Geometry: see drawing. Coordinates: mm, zero at the bounding-box minimum. A direction names the side the tool comes from. Give positions to 0.01 mm unless a question says otherwise; leave off trailing zeros. Loops run counter-clockwise (first coordinate to the right, second up) from the corner with the lowest first, then second, coordinate; pieces in that order, holes last. Notation, with made-up numbers: (56.25, 46) - (86.25, 46) arc R27 cw to (86.25, 82) - close; hole circle Ø5 at (50, 34.5). An arc over 180 degrees is marked (long way). Use one line per item in the form item = value.
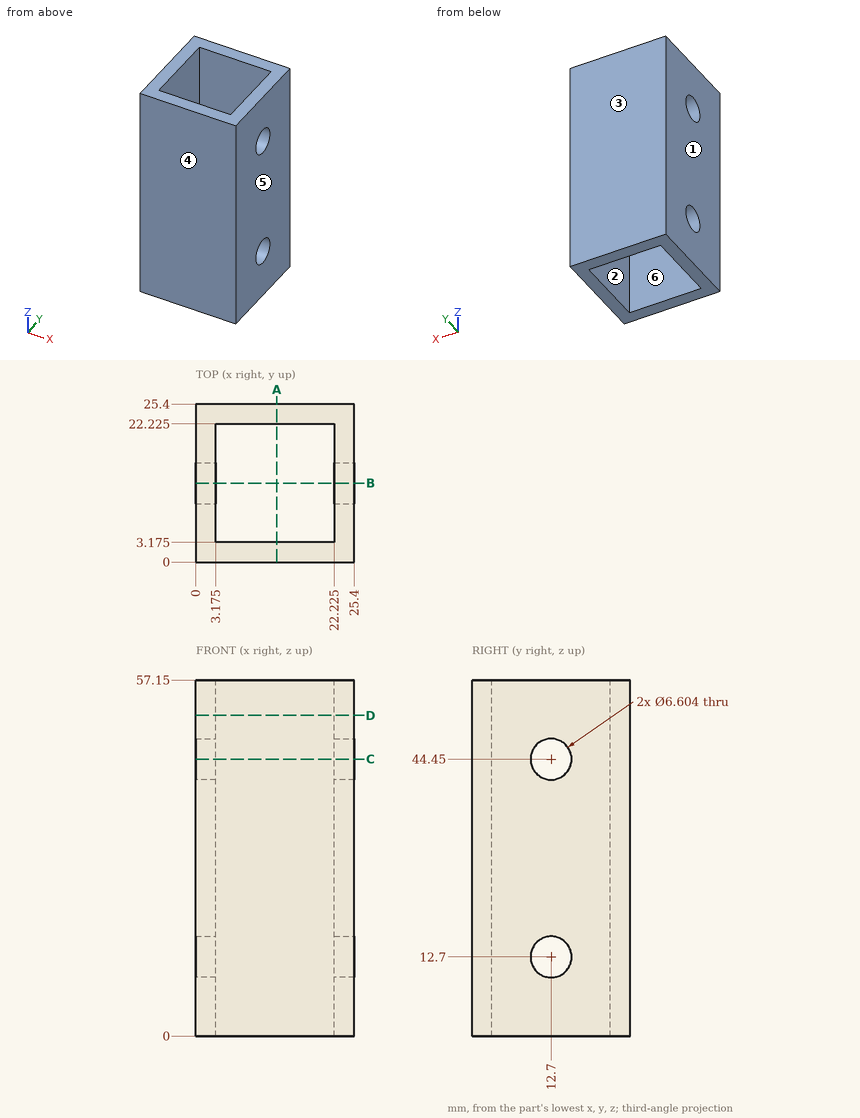
(1) Cut plane B-B (y = 12.7). Return the cut outline in (x, z) (3 decimals).
Solution:
outline = (0, 0) - (3.175, 0) - (3.175, 9.398) - (0, 9.398) - close; (0, 16.002) - (3.175, 16.002) - (3.175, 41.148) - (0, 41.148) - close; (0, 47.752) - (3.175, 47.752) - (3.175, 57.15) - (0, 57.15) - close; (22.225, 0) - (25.4, 0) - (25.4, 9.398) - (22.225, 9.398) - close; (22.225, 16.002) - (25.4, 16.002) - (25.4, 41.148) - (22.225, 41.148) - close; (22.225, 47.752) - (25.4, 47.752) - (25.4, 57.15) - (22.225, 57.15) - close
(2) Access query for the marked faces 5 and 6. Directions: +Z, -Z, +X, -X, +Y, -Y. A direction counts if a zero-diameter tool reaches every point of the face in a straight line with its end or side. Return the directions, or none.
Solution:
face_5 = +Z, -Z, +X, +Y, -Y
face_6 = +Z, -Z
(3) Cut plane A-A (x = 13). Return the cut outline in (y, z) (3 decimals), plus the area to 3 significant figures.
Solution:
outline = (0, 0) - (3.175, 0) - (3.175, 57.15) - (0, 57.15) - close; (22.225, 0) - (25.4, 0) - (25.4, 57.15) - (22.225, 57.15) - close
area = 363 mm2
(4) Material intervals for L1, parallel to Y at x = 16.5, z = 4 (3 decimals); L2, parallel to Y at x = 2.3, z = 12.7, sorted ascending. Write a range as from..to.
Solution:
L1 = 0..3.175, 22.225..25.4
L2 = 0..9.4, 16..25.4
(5) Cut plane C-C (z = 44.45). Return the cut outline in (x, y) (3 decimals).
Solution:
outline = (0, 0) - (25.4, 0) - (25.4, 9.398) - (22.225, 9.398) - (22.225, 3.175) - (3.175, 3.175) - (3.175, 9.398) - (0, 9.398) - close; (0, 16.002) - (3.175, 16.002) - (3.175, 22.225) - (22.225, 22.225) - (22.225, 16.002) - (25.4, 16.002) - (25.4, 25.4) - (0, 25.4) - close
(6) Pull-direction query (Y, two-part tool) for the marked faces 1, 2, 3 and 4; classes: released by +Y, released by -Y, zero draft, split by the parting line, or undercut.
Solution:
face_1 = zero draft
face_2 = undercut
face_3 = released by +Y
face_4 = released by -Y
(7) Cut plane D-D (z = 51.5). Return the cut outline in (x, y) (3 decimals).
Solution:
outline = (0, 0) - (25.4, 0) - (25.4, 25.4) - (0, 25.4) - close; hole (3.175, 3.175) - (22.225, 3.175) - (22.225, 22.225) - (3.175, 22.225) - close
